Work out the finished part from the listing and answer in its coordinate system (mm). Face numbers are marked on the shaded views. A direction names the side the tool comes from. Give positions to 0.01 mm unless a question says otherwise; leave off trailing zeros. Order: outer loops, then holes, each group sorted by start corner. A loop starts at its lowest first (then second) coordinate and runs counter-clockwise, first axis right, second up. Notation, with made-up numbers: (-7.5, -16) -> (18.5, -16) arc R34 cw to (18.5, 18) -> close; hole circle Ø3 at (9, 79). An arc over 180 degrees is marked (long way). Answer as CSV lines item,"result". Start each with the question number.
1. A cutting plane is placed at C-C (y = 4). Give the vertices of the cut face in (x, z), then the cut area to 3 significant figures.
2. A cutting plane is placed at A-A (z = -1.25). Give the vertices of the cut face in (x, y), then the cut area to 3 significant figures.
3. For a pull along Z with two mould halves and no side action, classify the marked faces 5, 6 and 7 as released by +Z, released by -Z, zero draft, split by the parting line, or undercut.
4. Find the intervals of material crossed by L1, parallel to Z at x = 3.5, y = 9; L2, parallel to Z at x = 3.5, y = 20; L3, parallel to Y at x = -1, z = 1, in increasing order.
5. A cutting plane is placed at B-B (x = 1.5). Give the vertices of the cut face in (y, z).
6. Flat-ended cylindrical pins translate along their axes: pin 1 (1 mm diameter, centred on x = 2, z = 1, fed in from -Y); pin 2 (2.5 mm diameter, centred on x = -1.5, y = 5, fed in from -Z); pin 3 (2.5 mm diameter, centred on x = 2.5, z = 3.5, fed in from +Y). Find the tip coordinate at first contact, or state that the pin passes through.
7. For the marked faces 1, 2, 3 and 4, determine the directions among +Z, -Z, +X, -X, +Y, -Y from which every point of the face is accessible in a straight line to the end or side of a thin tool.
8. A cutting plane is placed at D-D (x = -0.5). Give the vertices of the cut face in (y, z), then the cut area to 3 significant figures.
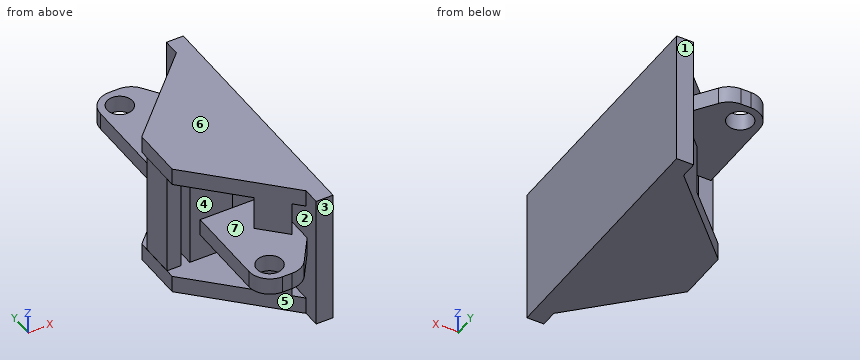
from build123d import *

# Parameters (mm, degrees)
F1_DEPTH      = 8
F1_DEPTH_BACK = 8
F2_W          = 11
F2_H          = 12
F3_DEPTH      = 30.001
F4_R          = 1.5
F5_DEPTH      = 2
F6_R          = 2.5
F8_DEPTH      = 16
F9_W          = 5.021157
F9_H          = 4
F9_W_2        = 1.667027
F10_DEPTH     = 12


with BuildPart() as f1:
    # F0 (on Top) → F1 (new body, two sides)
    with BuildSketch(Plane.XY) as f1_sk:
        Polygon((-5.6634, 11.949274), (6.285874, 0), (6.285874, 30), (-5.6634, 18.050726), align=None)
    extrude(amount=F1_DEPTH)
    extrude(f1_sk.sketch, amount=-F1_DEPTH_BACK)

    # F2 (on Front) → F3 (cut, through all)
    with BuildSketch(Plane.XZ):
        with Locations((-1.214126, 0)):
            Rectangle(F2_W, F2_H)
    extrude(amount=-F3_DEPTH, mode=Mode.SUBTRACT)

    # F4 (on Top) → F5 (join)
    with BuildSketch(Plane.XY):
        Polygon((4.371856, 9.871843), (-3.585968, 9.871843), (-3.585968, -2.374122), (1.36807, -2.374122), (4.371856, 1.914018), align=None)
        with Locations((-1.214126, 0)):
            Circle(F4_R, mode=Mode.SUBTRACT)
        Polygon((-3.585968, 20.128157), (4.371856, 20.128157), (4.371856, 28.085982), (1.36807, 32.374122), (-3.585968, 32.374122), align=None)
        with Locations((-1.214126, 30)):
            Circle(F4_R, mode=Mode.SUBTRACT)
    extrude(amount=F5_DEPTH)

    # F6
    f6_edges = [f1.edges().sort_by_distance(p)[0] for p in [
        (-3.585968, -2.374122, 1),
        (1.36807, -2.374122, 1),
        (-3.585968, 32.374122, 1),
        (1.36807, 32.374122, 1),
    ]]
    fillet(f6_edges, radius=F6_R)

    # F7 (on face) → F8 (join, through all)
    with BuildSketch(Plane.XY.offset(8)):
        Polygon((4.285874, 0), (6.285874, 0), (4.285874, 2), align=None)
        Polygon((4.285874, 28), (6.285874, 30), (4.285874, 30), align=None)
    extrude(amount=-F8_DEPTH)

    # F9 (on face) → F10 (join, through all)
    with BuildSketch(Plane.XY.offset(-6)):
        with Locations((-0.463468, 15)):
            Rectangle(F9_W, F9_H)
        with Locations((-4.812499, 15)):
            Rectangle(F9_W_2, F9_H)
        Polygon((3.246619, 24.120981), (3.246619, 26.960745), (0.406855, 24.120981), align=None)
        Polygon((0.406855, 5.879019), (3.246619, 3.039255), (3.246619, 5.879019), align=None)
    extrude(amount=F10_DEPTH)


solid = f1.part
Answer sheet:
1,outline,"(-3.59, 0) -> (2.29, 0) -> (2.29, -8) -> (6.29, -8) -> (6.29, 8) -> (2.29, 8) -> (2.29, 2) -> (-3.59, 2) -> close; hole (3.25, -6) -> (4.29, -6) -> (4.29, 0) -> (3.25, 0) -> close; hole (3.25, 2) -> (4.29, 2) -> (4.29, 6) -> (3.25, 6) -> close"
1,area,"65.4 mm^2"
2,outline,"(-5.65, 13) -> (-3.98, 13) -> (-3.98, 17) -> (-5.65, 17) -> close; (-2.97, 13) -> (2.05, 13) -> (2.05, 17) -> (-2.97, 17) -> close; (0.41, 5.88) -> (3.25, 3.04) -> (3.25, 5.88) -> close; (0.41, 24.12) -> (3.25, 24.12) -> (3.25, 26.96) -> close; (4.29, 0) -> (6.29, 0) -> (6.29, 30) -> (4.29, 30) -> close"
2,area,"94.8 mm^2"
3,face 5,"zero draft"
3,face 6,"released by +Z"
3,face 7,"undercut"
4,L1,"z = -8 to -6, 0 to 2, 6 to 8"
4,L2,"z = -8 to -6, 6 to 8"
4,L3,"y = -2.37 to -1.48, 1.48 to 9.87, 13 to 17, 20.13 to 28.52, 31.48 to 32.37"
5,outline,"(-1.92, 0) -> (4.79, 0) -> (4.79, -8) -> (25.21, -8) -> (25.21, 0) -> (31.92, 0) -> (31.92, 2) -> (25.21, 2) -> (25.21, 8) -> (4.79, 8) -> (4.79, 2) -> (-1.92, 2) -> close; hole (5.88, -6) -> (13, -6) -> (13, 6) -> (5.88, 6) -> (5.88, 2) -> (9.87, 2) -> (9.87, 0) -> (5.88, 0) -> close; hole (17, -6) -> (24.12, -6) -> (24.12, 0) -> (20.13, 0) -> (20.13, 2) -> (24.12, 2) -> (24.12, 6) -> (17, 6) -> close"
6,pin 1,"stops at y = -1.92"
6,pin 2,"stops at z = 0"
6,pin 3,"stops at y = 26.96"
7,face 1,"+Z, -Z, +X, +Y"
7,face 2,"none"
7,face 3,"+Z, -Z, +X, -Y"
7,face 4,"-X"
8,outline,"(-2.37, 0) -> (-1.32, 0) -> (-1.32, 2) -> (-2.37, 2) -> close; (1.32, 0) -> (9.87, 0) -> (9.87, 2) -> (1.32, 2) -> close; (6.79, -8) -> (23.21, -8) -> (23.21, -6) -> (17, -6) -> (17, 6) -> (23.21, 6) -> (23.21, 8) -> (6.79, 8) -> (6.79, 6) -> (13, 6) -> (13, -6) -> (6.79, -6) -> close; (20.13, 0) -> (28.68, 0) -> (28.68, 2) -> (20.13, 2) -> close; (31.32, 0) -> (32.37, 0) -> (32.37, 2) -> (31.32, 2) -> close"
8,area,"152 mm^2"
